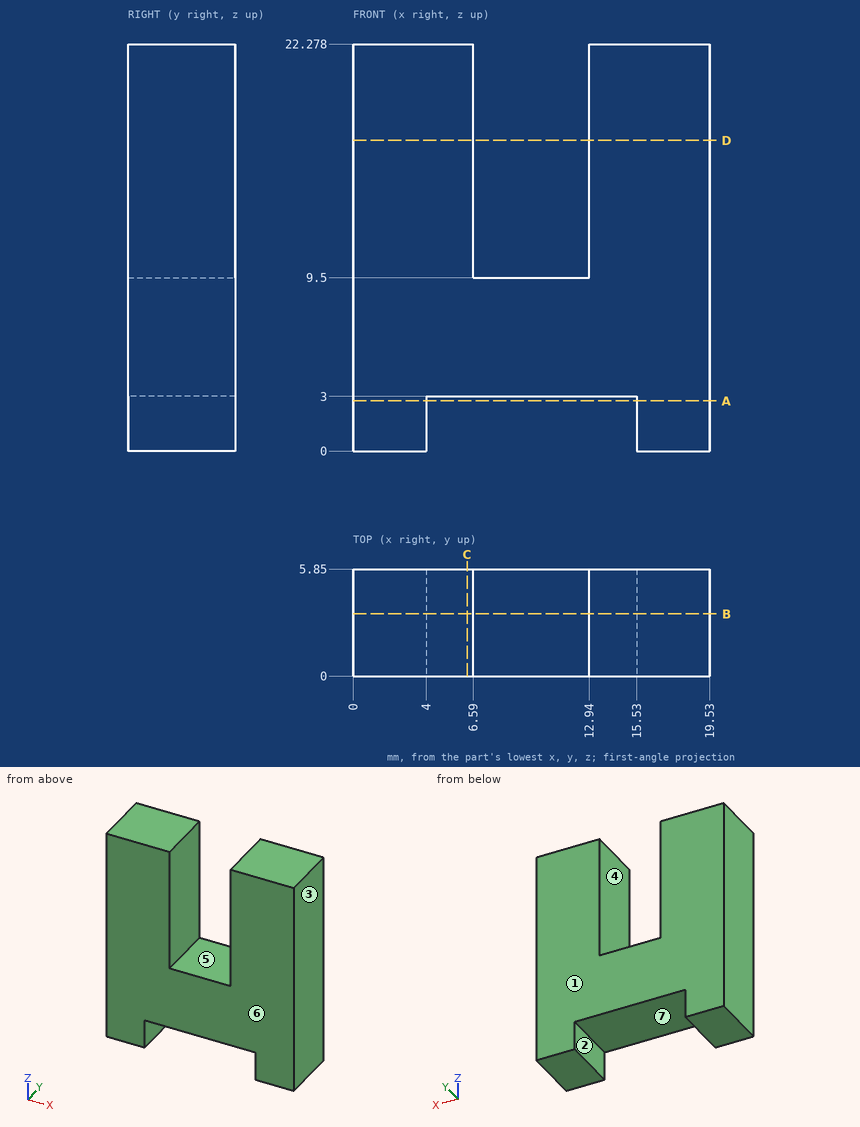
Check sheet for the drawn part. Datum: minimum x, y, z corner. Units: mm. A direction names the side the tool comes from. Round coordinates to 2 decimals unless told otherwise and drop trailing zeros. Loops run counter-clockwise (first coordinate to the right, second up) from the corner with the lowest first, then second, coordinate; pieces in that order, holes last. Notation, with made-up numbers: (78, 67.25) - (101, 67.25) arc R18 ccw to (101, 77.25) - close; hole circle Ø8 at (59, 38.5). An arc over 180 degrees is marked (long way). Answer as a JSON object with one key per item and string values. Group by question number.
Q1. Mould release check, pull along X, two halves, no side actions. Record for the marked faces 1, 2, 3 and 4: released by +X, released by -X, zero draft, split by the parting line, or undercut.
Q2. Sectioned sample at C-C, the plane x = 6.25. Enter the section's corners in (y, z), plus the area to 3 significant figures.
Q3. Scan lines: line 1 along X through (y, z) = (2.5, 14.5); line 2 along X through (y, z) = (5.35, 2.5); line 3 along Z through (x, y) = (8, 2.6). Record each from-to range of solid material in increasing order. Write a range as [from, to].
Q4. Sectioned sample at B-B, the plane y = 3.4. Enter the section's corners in (x, z).
Q5. Sectioned sample at D-D, the plane z = 17. Enter the section's corners in (x, y), plus the area to 3 significant figures.
Q6. Sectioned sample at A-A, the plane z = 2.75. Enter the section's corners in (x, y).
Q7. Set-up check for the marked faces 5, 6 and 7: record each of +Z, -Z, +X, -X, +Y, -Y from which the full face is reachable in a straight line by a thin tool's end or side.
Solution:
{
 "1": {"face 1": "zero draft", "face 2": "undercut", "face 3": "released by +X", "face 4": "undercut"},
 "2": {"outline": "(0, 3) - (5.85, 3) - (5.85, 22.28) - (0, 22.28) - close", "area": "113 mm²"},
 "3": {"line 1": "x = [0, 6.59], [12.94, 19.53]", "line 2": "x = [0, 4], [15.53, 19.53]", "line 3": "z = [3, 9.5]"},
 "4": {"outline": "(0, 0) - (4, 0) - (4, 3) - (15.53, 3) - (15.53, 0) - (19.53, 0) - (19.53, 22.28) - (12.94, 22.28) - (12.94, 9.5) - (6.59, 9.5) - (6.59, 22.28) - (0, 22.28) - close"},
 "5": {"outline": "(0, 0) - (6.59, 0) - (6.59, 5.85) - (0, 5.85) - close; (12.94, 0) - (19.53, 0) - (19.53, 5.85) - (12.94, 5.85) - close", "area": "77.1 mm²"},
 "6": {"outline": "(0, 0) - (4, 0) - (4, 5.85) - (0, 5.85) - close; (15.53, 0) - (19.53, 0) - (19.53, 5.85) - (15.53, 5.85) - close"},
 "7": {"face 5": "+Z, +Y, -Y", "face 6": "+Z, -Z, +X, -X, -Y", "face 7": "-Z, +Y, -Y"}
}
